The model under review builds one solid part; all positions refer to its coordinate system, in mm. A direction names the side the tool comes from. Coordinates: 2 decimals unless noted, no trailing zeros. Order: outer loops, then holes, each group sorted by start corner. A loop starts at its lowest first (then second) coordinate and runs counter-clockwise, first axis right, second up. Notation, with made-up numbers: M 24.5,48 L 66.5,48 A16 ccw 66.5,66 Z; hole C 32.25,2.5 d4. An arc over 180 degrees is marked long. Answer in a Markdown table with one row per item.
Autodesk Inventor part; units mm, degrees
ref_plane "YZ Plane" through (0, 0, 0) normal (1, 0, 0) x (0, 1, 0)
ref_plane "XZ Plane" through (0, 0, 0) normal (0, 1, 0) x (-1, 0, 0)
ref_plane "XY Plane" through (0, 0, 0) normal (0, 0, 1) x (1, 0, 0)
sketch "Sketch1" plane through (0, 0, 0) normal (0, 0, 1) x (1, 0, 0)
  line L0 (0, 0) -> (35.7, 0)
  line L1 (35.7, 0) -> (35.7, 30.8)
  line L2 (35.7, 30.8) -> (0, 30.8)
  line L3 (0, 30.8) -> (0, 0)
  dimension "d0" = 35.7
  dimension "d1" = 30.8
extrude "Extrusion1" add sketch "Sketch1" along normal blind 6
sketch "Sketch4" plane through (0, 0, 6) normal (0, 0, 1) x (1, 0, 0)
  line L0 (35.7, 30.8) -> (0, 30.8)
  line L1 (35.7, 0) -> (32.7, 0)
  line L2 (32.7, 0) -> (32.7, 30.8)
  line L3 (32.7, 30.8) -> (35.7, 30.8)
  line L4 (35.7, 30.8) -> (35.7, 0)
  point P0 (0, 0)
  dimension "d10" = 3
extrude "Extrusion3" add sketch "Sketch4" along normal blind 21.5
sketch "Sketch24" plane through (0, 30.8, 0) normal (0, 1, 0) x (1, 0, 0)
  line L0 (2, 15) -> (52.2252, 23.8561)
  line L1 (35.7, 0) -> (35.7, -27.5)
  line L2 (2, 15) -> (0, 0)
  line L3 (0, 0) -> (0, -6)
  line L4 (0, 0) -> (0, -6)
  line L5 (0, -6) -> (32.7, -6)
  line L6 (35.7, 0) -> (35.7, -27.5)
  line L7 (32.7, -6) -> (52.2252, 8)
  line L8 (52.2252, 23.8561) -> (52.2252, 8)
  line L9 (35.7, 0) -> (0, 0)
  circle A0 centre (45.2252, 19.9817) radius 0.5
  circle A1 centre (28.4835, 17.0296) radius 0.5
  circle A2 centre (11.7417, 14.0776) radius 0.5
  dimension "d152" = 51
  dimension "d153" = 80
  dimension "d155" = 15
  dimension "d159" = 17
  dimension "d160" = 1
  dimension "d161" = 1
  dimension "d162" = 2.6
  dimension "d163" = 2.6
  dimension "d164" = 7
  dimension "d165" = 2.6
  dimension "d166" = 17
  dimension "d167" = 2
  dimension "d168" = 8
  dimension "d169" = 1
extrude "Extrusion19" add sketch "Sketch24" along normal blind 3
ref_plane "Work Plane22" through (32.7, 15.4, 27.5) normal (0, 1, 0) x (1, 0, 0)
mirror "Mirror11" about plane through (32.7, 15.4, 27.5) normal (0, 1, 0) of "Extrusion19"
mirror "Mirror3" about plane through (34.2, 15.4, 27.5) normal (0, 0, 1) of "Extrusion1", "Extrusion3", "Extrusion19", "Mirror11"
sketch "Sketch28" plane through (35.7, 30.8, 51.1511) normal (0, 1, 0) x (1, 0, 0)
  circle A0 centre (-23.9583, -17.9266) radius 0.5
  circle A1 centre (-7.2165, -20.8786) radius 0.5
  circle A2 centre (9.5252, -23.8306) radius 0.5
  circle A3 centre (-23.9583, 65.2287) radius 0.5
  circle A4 centre (-7.2165, 68.1807) radius 0.5
  circle A5 centre (9.5252, 71.1327) radius 0.5
  line L0 (-35.7, 51.1511) -> (-33.7, 66.1511)
  line L1 (-33.7, 66.1511) -> (16.5252, 75.0071)
  line L2 (16.5252, 75.0071) -> (16.5252, 59.1511)
  line L3 (16.5252, 59.1511) -> (0, 47.3021)
  line L4 (0, 47.3021) -> (-3, 45.1511)
  line L5 (-3, 2.1511) -> (-3, 45.1511)
  line L6 (-3, 2.1511) -> (0, 0)
  line L7 (0, 47.3021) -> (0, 0)
  line L8 (-35.7, 51.1511) -> (0, 51.1511)
  line L9 (-35.7, 45.1511) -> (-35.7, 51.1511)
  line L10 (-3, 45.1511) -> (-35.7, 45.1511)
  line L11 (0, 51.1511) -> (0, 47.3021)
  line L12 (-35.7, 2.1511) -> (-3, 2.1511)
  line L13 (-35.7, -3.8489) -> (-35.7, 2.1511)
  line L14 (0, -3.8489) -> (-35.7, -3.8489)
  line L15 (0, 0) -> (0, -3.8489)
  line L16 (0, 0) -> (16.5252, -11.8489)
  line L17 (16.5252, -11.8489) -> (16.5252, -27.705)
  line L18 (16.5252, -27.705) -> (-33.7, -18.8489)
  line L19 (-33.7, -18.8489) -> (-35.7, -3.8489)
  line L20 (0, 47.3021) -> (0, 0)
  line L21 (0, 8.2511) -> (-3, 8.2511)
  line L22 (-3, 8.2511) -> (-3, 39.0511)
  line L23 (-3, 39.0511) -> (0, 39.0511)
  line L24 (0, 39.0511) -> (0, 8.2511)
  point P0 (-3, 23.6511)
  point P1 (-3, 23.6511)
  dimension "d205" = 30.8
  dimension "d206" = 3
extrude "Extrusion21" add sketch "Sketch28" along normal blind 23 contours L7 L21 L5 L23
sketch "Sketch29" plane through (32.7, 0, 6) normal (-1, 0, 0) x (0, 0, 1)
  line L0 (36.9, 30.8) -> (36.9, 53.8)
  line L1 (6.1, 33.8) -> (36.9, 33.8)
  line L2 (36.9, 33.8) -> (36.9, 36.8)
  line L3 (36.9, 36.8) -> (6.1, 36.8)
  line L4 (6.1, 36.8) -> (6.1, 33.8)
  line L5 (6.1, 53.8) -> (36.9, 53.8)
  line L6 (6.1, 30.8) -> (6.1, 53.8)
  point P0 (-6, 0)
  dimension "d207" = 3
  dimension "d208" = 17
extrude "Extrusion22" add sketch "Sketch29" along normal blind 36.1 contours L1 L4 L3 L0
sketch "Sketch30" plane through (-3.4, 0, 6) normal (-1, 0, 0) x (0, 0, 1)
  line L0 (6.1, 36.8) -> (36.9, 36.8)
  line L1 (36.9, 36.8) -> (36.9, 53.8)
  line L2 (6.1, 53.8) -> (36.9, 53.8)
  line L3 (6.1, 36.8) -> (6.1, 53.8)
  line L4 (6.1, 33.8) -> (36.9, 33.8)
  line L5 (36.9, 33.8) -> (36.9, 36.8)
  line L6 (36.9, 36.8) -> (6.1, 36.8)
  line L7 (6.1, 36.8) -> (6.1, 33.8)
  point P0 (-6, 0)
extrude "Extrusion23" add sketch "Sketch30" along normal blind 3
sketch "Sketch31" plane through (32.7, 30.8, 42.9) normal (0, 0, 1) x (1, 0, 0)
  line L0 (-39.1, 3) -> (3, 3)
  line L1 (3, 3) -> (3, 23)
  line L2 (3, 23) -> (-39.1, 23)
  line L3 (-39.1, 23) -> (-39.1, 3)
  circle A0 centre (-32.9, 15.3) radius 0.5
  circle A1 centre (-26.55, 8.875) radius 0.5
  circle A2 centre (-9.55, 8.875) radius 0.5
  circle A3 centre (-3.2, 15.3) radius 0.5
  line L4 (-32.9, 15.3) -> (-3.2, 15.3) construction
  line L5 (-26.55, 8.875) -> (-9.55, 8.875) construction
  line L6 (0, 6) -> (-36.1, 6) construction
  line L7 (-30.55, 23) -> (-5.55, 23)
  line L8 (-5.55, 23) -> (-5.55, 11.25)
  line L9 (-5.55, 11.25) -> (-30.55, 11.25)
  line L10 (-30.55, 11.25) -> (-30.55, 23)
  point P0 (-32.7, -30.8)
  point P1 (-18.05, 15.3)
  point P2 (-18.05, 23)
  point P3 (-18.05, 8.875)
  point P4 (-18.05, 11.25)
  dimension "d211" = 1
  dimension "d212" = 17
  dimension "d213" = 29.7
  dimension "d214" = 2.875
  dimension "d215" = 9.3
  dimension "d216" = 5.25
  dimension "d217" = 25
extrude "Extrusion24" add sketch "Sketch31" along normal blind 3 contours L3 L2 L10 L9 L8 L1 L0
ref_plane "Work Plane23" through (32.7, 0, 27.5) normal (0, 0, 1) x (1, 0, 0)
mirror "Mirror13" about plane through (32.7, 0, 27.5) normal (0, 0, 1) of "Extrusion24"
sketch "Sketch32" plane through (35.7, 30.8, 3.8489) normal (1, 0, 0) x (0, 0, -1)
  line L0 (3.8489, -30.8) -> (3.8489, 0)
  line L1 (3.8489, 0) -> (0, 0)
  line L2 (0, 0) -> (-8.2511, 0)
  line L3 (-8.2511, 0) -> (-8.2511, 3)
  line L4 (-8.2511, 3) -> (-5.2511, 3)
  line L5 (-5.2511, 3) -> (-5.2511, 23)
  line L6 (-5.2511, 23) -> (-42.0511, 23)
  line L7 (-42.0511, 3) -> (-42.0511, 23)
  line L8 (-39.0511, 3) -> (-42.0511, 3)
  line L9 (-39.0511, 0) -> (-39.0511, 3)
  line L10 (-39.0511, 0) -> (-47.3021, 0)
  line L11 (-51.1511, 0) -> (-47.3021, 0)
  line L12 (-51.1511, -30.8) -> (-51.1511, 0)
  line L13 (-47.3021, -30.8) -> (-51.1511, -30.8)
  line L14 (0, -30.8) -> (-47.3021, -30.8)
  line L15 (3.8489, -30.8) -> (0, -30.8)
  line L16 (-39.0511, 0) -> (-45.1511, 0)
  line L17 (-45.1511, 0) -> (-45.1511, 3)
  line L18 (-45.1511, 3) -> (-39.0511, 3)
  line L19 (-39.0511, 3) -> (-39.0511, 0)
  line L20 (-8.2511, 0) -> (-2.1511, 0)
  line L21 (-2.1511, 0) -> (-2.1511, 3)
  line L22 (-2.1511, 3) -> (-8.2511, 3)
  line L23 (-8.2511, 3) -> (-8.2511, 0)
extrude "Extrusion25" add sketch "Sketch32" against normal up to surface (35.7 mm away) contours L2 L3 L4 L22 L21 | L17 L18 L8 L9 L10
chamfer "Chamfer9" distance 2 angle 45 2 edges at (16.35, 30.8, 12.1) (16.35, 30.8, 42.9)
sketch "Sketch33" plane through (32.7, 30.8, 49) normal (0, 1, 0) x (1, 0, 0)
  line L0 (3, 0) -> (3, -2.1511)
  line L1 (3, 0) -> (0, 0)
  line L2 (3, -2.1511) -> (0, 0)
  line L3 (3, 45.1511) -> (0, 43)
  line L4 (3, 45.1511) -> (3, 43)
  line L5 (0, 43) -> (3, 43)
  point P0 (-32.7, 49)
extrude "Extrusion26" add sketch "Sketch33" along normal up to surface (3 mm away)
chamfer "Chamfer10" distance 2 angle 45 5 edges at (-6.4, 33.8, 27.5) (-3.2, 33.8, 45.9) (-6.4, 43.8, 45.9) (-3.2, 33.8, 9.1) (-6.4, 43.8, 9.1)
ref_plane "Work Plane3" through (17.85, 0, 49) normal (-1, 0, 0) x (0, 1, 0)
ref_plane "Work Plane4" through (35.7, 10.55, 49) normal (0, -1, 0) x (-1, 0, 0)
properties part number "RearConnector"
(1) Insertion check: P1, Ø8, axis at y = 25.5, z = 56, coming from the +X side; P2, Ø9.5, axis at y = 15, z = 48, coming from the -X side; P3, Ø4, axis at y = 7, z = 26, coming from the -X side; P4, Ø5, axis at x = 13.5, y = 45.5, coming from the -Z side. Each pin has a flat end and moves straight along its axis. Give the tip position at first contact, or say it passes through.
Report:
| item | result |
|---|---|
| P1 | x = 35.7 |
| P2 | x = 0 |
| P3 | x = 32.7 |
| P4 | through |
(2) Machinability: for faces 1 (the flat face through (18, 16, 55)), 2 (the flat face through (32.7, 17, 28)), 3 (the flat face through (26, 33.8, -7)), 4 (the flat face through (15, 36.8, 28)), 5 (the flat face through (2.15, 48, 44)), which of the approach directions +Z, -Z, +X, -X, +Y, -Y give a long, thin tool a straight path to every point of the face, cutting with its end or side? Answer none if there is none.
Report:
| item | result |
|---|---|
| face 1 | +Z, +X, -X |
| face 2 | -X, -Y |
| face 3 | -Z, +X, -X, +Y |
| face 4 | +Y |
| face 5 | +Z, -Z, +Y |
(3) The part is to be moulded in two halves that separate along X. For faces 6 (the flat face through (-5.4, 34.8, 27.3)), 7 (the flat face through (27.15, 48, 44)), 8 (the flat face through (-4, 53.8, 28)), say which applies: +X half, -X half, draft (parallel to the pull), parting line (faces both ways), or undercut.
Report:
| item | result |
|---|---|
| face 6 | -X half |
| face 7 | undercut |
| face 8 | draft |
(4) Take a section at D-D (z = 31.5). Write out the cut boundary in (x, y).
Report:
| item | result |
|---|---|
| outline | M -6.4,35.8 L -4.4,33.8 L 32.7,33.8 L 32.7,0 L 35.7,0 L 35.7,53.8 L 32.7,53.8 L 32.7,36.8 L -3.4,36.8 L -3.4,53.8 L -6.4,53.8 Z |
(5) Take a section at B-B (x = 47). Write out the cut boundary in (y, z), then the cut area to 3 significant figures.
Report:
| item | result |
|---|---|
| outline | M -3,-22.93 L 0,-22.93 L 0,-4.25 L -3,-4.25 Z; M -3,59.25 L 0,59.25 L 0,77.93 L -3,77.93 Z; M 30.8,-22.93 L 33.8,-22.93 L 33.8,-4.25 L 30.8,-4.25 Z; M 30.8,59.25 L 33.8,59.25 L 33.8,77.93 L 30.8,77.93 Z |
| area | 224 mm^2 |
(6) Take a section at C-C (y = 6). Write out the cut boundary in (x, z), then the cut area to 3 significant figures.
Report:
| item | result |
|---|---|
| outline | M 0,0 L 35.7,0 L 35.7,55 L 0,55 L 0,49 L 32.7,49 L 32.7,6 L 0,6 Z |
| area | 557 mm^2 |
(7) Take a section at A-A (z = 65.5). Write out the cut boundary in (x, y).
Report:
| item | result |
|---|---|
| outline | M 1.4,-3 L 52.23,-3 L 52.23,0 L 1.4,0 Z; M 1.4,30.8 L 52.23,30.8 L 52.23,33.8 L 1.4,33.8 Z |
(8) To check wall thickness, follow line 1 (Z direction, x = 2, y = 14); line 2 (Y direction, x = 43.5, z = -10.5); line 3 (X direction, y = 46, z = 35). State the ranges of each line that lie inside material, in increasing order. Write a range as [from, to].
Report:
| item | result |
|---|---|
| line 1 | [0, 6], [49, 55] |
| line 2 | [-3, 0], [30.8, 33.8] |
| line 3 | [-6.4, -3.4], [32.7, 35.7] |
